The model under review builds one solid part; all positions refer to its coordinate system, in mm. Round coordinates to 2 decimals unless told otherwise and drop trailing zeros. Return JSON: item names as keys, results as strings.
from build123d import *

# Parameters (mm, degrees)
SKETCH1_R        = 2.2
SKETCH1_R_2      = 1.85915493
SKETCH1_R_3      = 1.8
SKETCH1_R_4      = 1.35
SKETCH1_R_5      = 1.983111479
EXTRUSION1_DEPTH = 1.6
FILLET1_R        = 1
FILLET2_R        = 4
FILLET3_R        = 3
FILLET4_R        = 3
FILLET5_R        = 2
FILLET6_R        = 2
FILLET7_R        = 3
FILLET8_R        = 3
FILLET9_R        = 2
FILLET10_R       = 2
FILLET11_R       = 3


with BuildPart() as part:
    # Sketch1 → Extrusion1 (new body)
    with BuildSketch(Plane(origin=(0, 0, 0), x_dir=(-1, 0, 0), z_dir=(0, 1, 0))):
        Polygon((74.087520418, 321.088295015), (70.369210559, 327.285477572), (45.580478165, 327.285477572), (45.580478165, 312.412238135), (23.246043749, 290.934342561), (26.682507041, 287.360833055), (12.735407819, 253.538985229), (9.017097883, 253.538985229), (9.017097883, 226.891111382), (9.017097883, 200.243237534), (12.735407819, 200.243237534), (26.682507041, 166.421389708), (23.246043749, 162.847880202), (45.580478165, 141.369984628), (45.580478165, 126.496745191), (70.369210559, 126.496745191), (74.087520418, 132.693927748), (97.636816193, 132.693927748), (121.186111968, 132.693927748), (124.904421827, 126.496745191), (149.693154221, 126.496745191), (149.693154221, 141.369984628), (172.027588636, 162.847880202), (168.591125345, 166.421389708), (182.538224567, 200.243237534), (186.256534503, 200.243237534), (186.256534503, 226.891111382), (186.256534503, 253.538985229), (182.538224567, 253.538985229), (168.591125345, 287.360833055), (172.027588636, 290.934342561), (149.693154221, 312.412238135), (149.693154221, 327.285477572), (124.904421827, 327.285477572), (121.186111968, 321.088295015), (97.636816193, 321.088295015), align=None)
        with Locations((112.636816193, 211.891111382)):
            Circle(SKETCH1_R, mode=Mode.SUBTRACT)
        with Locations((49.266182018, 151.62213525)):
            Circle(SKETCH1_R_2, mode=Mode.SUBTRACT)
        with Locations((112.636816193, 241.891111382)):
            Circle(SKETCH1_R, mode=Mode.SUBTRACT)
        with Locations((82.636816193, 241.891111382)):
            Circle(SKETCH1_R, mode=Mode.SUBTRACT)
        with Locations((82.636816193, 211.891111382)):
            Circle(SKETCH1_R, mode=Mode.SUBTRACT)
        with Locations((176.256534503, 218.641111382)):
            Circle(SKETCH1_R_3, mode=Mode.SUBTRACT)
        with Locations((176.256534503, 235.141111382)):
            Circle(SKETCH1_R_3, mode=Mode.SUBTRACT)
        with Locations((19.017097883, 218.641111382)):
            Circle(SKETCH1_R_3, mode=Mode.SUBTRACT)
        with Locations((19.017097883, 235.141111382)):
            Circle(SKETCH1_R_3, mode=Mode.SUBTRACT)
        with Locations((182.756534503, 215.891111382)):
            Circle(SKETCH1_R_4, mode=Mode.SUBTRACT)
        with Locations((181.918506411, 237.891111382)):
            Circle(SKETCH1_R_4, mode=Mode.SUBTRACT)
        with Locations((51.777661187, 316.130534525)):
            Circle(SKETCH1_R_2, mode=Mode.SUBTRACT)
        with Locations((49.266182018, 302.160087513)):
            Circle(SKETCH1_R_2, mode=Mode.SUBTRACT)
        with Locations((13.355125975, 237.891111382)):
            Circle(SKETCH1_R_4, mode=Mode.SUBTRACT)
        with Locations((143.495971199, 137.651688238)):
            Circle(SKETCH1_R_2, mode=Mode.SUBTRACT)
        with Locations((146.007450368, 151.62213525)):
            Circle(SKETCH1_R_2, mode=Mode.SUBTRACT)
        with Locations((143.495971199, 316.130534525)):
            Circle(SKETCH1_R_2, mode=Mode.SUBTRACT)
        with Locations((146.007450368, 302.160087513)):
            Circle(SKETCH1_R_2, mode=Mode.SUBTRACT)
        with Locations((12.517097883, 215.891111382)):
            Circle(SKETCH1_R_4, mode=Mode.SUBTRACT)
        with Locations((51.777661187, 137.651688238)):
            Circle(SKETCH1_R_2, mode=Mode.SUBTRACT)
        with Locations((67.636816193, 196.891111382)):
            Circle(SKETCH1_R_5, mode=Mode.SUBTRACT)
        with Locations((67.636816193, 256.891111382)):
            Circle(SKETCH1_R_5, mode=Mode.SUBTRACT)
        with Locations((42.888078851, 158.000238416)):
            Circle(SKETCH1_R_2, mode=Mode.SUBTRACT)
        with Locations((152.385553534, 295.781984347)):
            Circle(SKETCH1_R_2, mode=Mode.SUBTRACT)
        with Locations((42.888078851, 295.781984347)):
            Circle(SKETCH1_R_2, mode=Mode.SUBTRACT)
        with Locations((127.636816193, 256.891111382)):
            Circle(SKETCH1_R_5, mode=Mode.SUBTRACT)
        with Locations((152.385553534, 158.000238416)):
            Circle(SKETCH1_R_2, mode=Mode.SUBTRACT)
        with Locations((127.636816193, 196.891111382)):
            Circle(SKETCH1_R_5, mode=Mode.SUBTRACT)
    extrude(amount=EXTRUSION1_DEPTH)

    # Fillet1
    fillet1_edges = [part.edges().sort_by_distance(p)[0] for p in [
        (-121.186111968, 0.8, 321.088295015),
        (-121.186111968, 0.8, 132.693927748),
        (-74.087520418, 0.8, 132.693927748),
        (-74.087520418, 0.8, 321.088295015),
    ]]
    fillet(fillet1_edges, radius=FILLET1_R)

    # Fillet2
    fillet2_edges = [part.edges().sort_by_distance(p)[0] for p in [
        (-149.693154221, 0.8, 327.285477572),
        (-149.693154221, 0.8, 126.496745191),
        (-45.580478165, 0.8, 126.496745191),
        (-45.580478165, 0.8, 327.285477572),
    ]]
    fillet(fillet2_edges, radius=FILLET2_R)

    # Fillet3
    fillet3_edges = [part.edges().sort_by_distance(p)[0] for p in [
        (-149.693154221, 0.8, 312.412238135),
        (-149.693154221, 0.8, 141.369984628),
        (-45.580478165, 0.8, 141.369984628),
        (-45.580478165, 0.8, 312.412238135),
    ]]
    fillet(fillet3_edges, radius=FILLET3_R)

    # Fillet4
    fillet4_edges = [part.edges().sort_by_distance(p)[0] for p in [
        (-172.027588636, 0.8, 290.934342561),
    ]]
    fillet(fillet4_edges, radius=FILLET4_R)

    # Fillet5
    fillet5_edges = [part.edges().sort_by_distance(p)[0] for p in [
        (-168.591125345, 0.8, 287.360833055),
    ]]
    fillet(fillet5_edges, radius=FILLET5_R)

    # Fillet6
    fillet6_edges = [part.edges().sort_by_distance(p)[0] for p in [
        (-26.682507041, 0.8, 287.360833055),
    ]]
    fillet(fillet6_edges, radius=FILLET6_R)

    # Fillet7
    fillet7_edges = [part.edges().sort_by_distance(p)[0] for p in [
        (-23.246043749, 0.8, 290.934342561),
    ]]
    fillet(fillet7_edges, radius=FILLET7_R)

    # Fillet8
    fillet8_edges = [part.edges().sort_by_distance(p)[0] for p in [
        (-172.027588636, 0.8, 162.847880202),
        (-23.246043749, 0.8, 162.847880202),
    ]]
    fillet(fillet8_edges, radius=FILLET8_R)

    # Fillet9
    fillet9_edges = [part.edges().sort_by_distance(p)[0] for p in [
        (-168.591125345, 0.8, 166.421389708),
        (-26.682507041, 0.8, 166.421389708),
    ]]
    fillet(fillet9_edges, radius=FILLET9_R)

    # Fillet10
    fillet10_edges = [part.edges().sort_by_distance(p)[0] for p in [
        (-182.538224567, 0.8, 253.538985229),
        (-182.538224567, 0.8, 200.243237534),
        (-12.735407819, 0.8, 200.243237534),
        (-12.735407819, 0.8, 253.538985229),
    ]]
    fillet(fillet10_edges, radius=FILLET10_R)

    # Fillet11
    fillet11_edges = [part.edges().sort_by_distance(p)[0] for p in [
        (-186.256534503, 0.8, 200.243237534),
        (-186.256534503, 0.8, 253.538985229),
        (-9.017097883, 0.8, 253.538985229),
        (-9.017097883, 0.8, 200.243237534),
    ]]
    fillet(fillet11_edges, radius=FILLET11_R)


solid = part.part
(1) Clearance check with a flat-ended pin moving along its axis: pin 1 Ø8 at (x, z) = (-165.5, 201) entering from -Y. State where the tip first meets the part, or that it passes through.
Filled in:
{"pin 1": "stops at y = 0"}
(2) Wall thickness on line 1 (Z direction, x = -67, y = 0.8); line 2 (X direction, y = 0.55, z = 295); line 3 (Z direction, x = -117.5, y = 0.5): over which ranges is each line inside the solid? List them lowest first.
Filled in:
{"line 1": "z = 126.5 to 195.01, 198.77 to 255.01, 258.77 to 327.29", "line 2": "x = -167.8 to -154.07, -150.7 to -44.57, -41.2 to -27.47", "line 3": "z = 132.69 to 321.09"}
(3) Mouldability with a two-part tool opening along Z and no side actions: class faces 1 (the flat face through (-34.9, 0.79, 151.64)), 2 (the flat face through (-160.374, 0.789, 302.141)), 3 (the cylindrical face through (-113.65, 0.79, 239.94)), 4 (the flat face through (-96, 1.6, 228)) as released by +Z, released by -Z, zero draft, split by the parting line, or undercut.
Filled in:
{"face 1": "released by -Z", "face 2": "released by +Z", "face 3": "undercut", "face 4": "zero draft"}
(4) Add section A-A (y = 1.1). Give the number of separate pieces and of enclosed holes in the cut face, plus the area to 3 significant figures.
Filled in:
{"separate pieces": "1", "enclosed holes": "28", "area": "28,600 mm2"}
